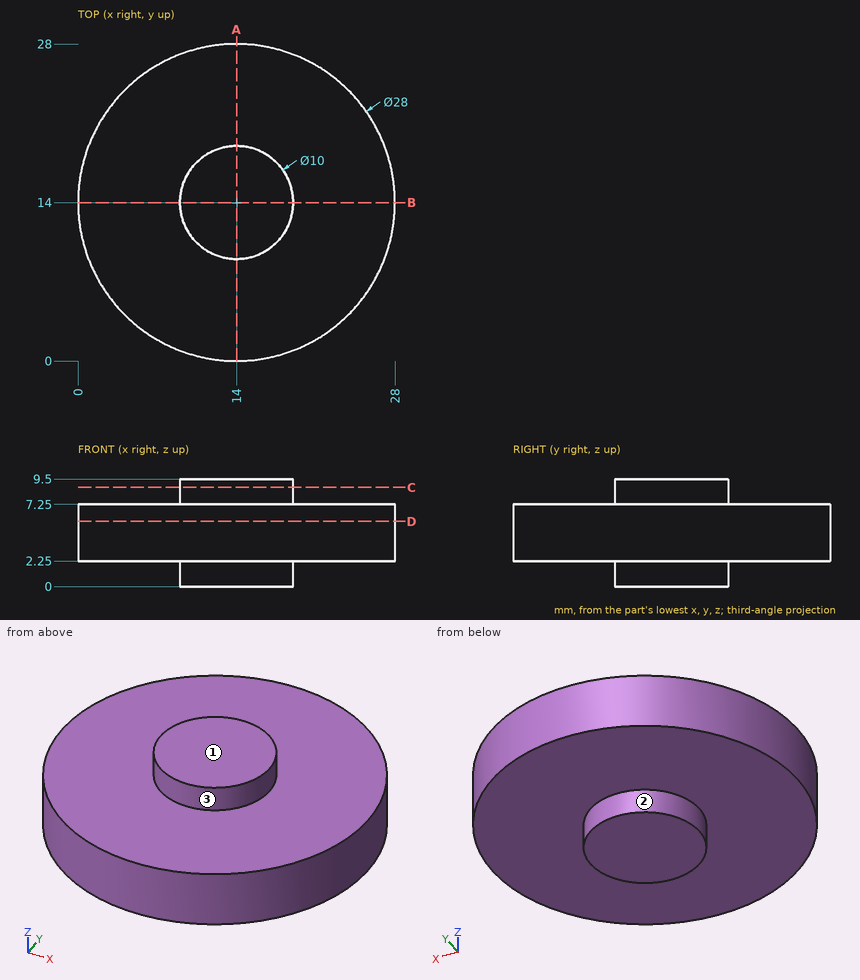
Could you check a few things on this drawing? It's one solid part, dimensions in mm from its lowest x, y, z. A direction names the side the tool comes from. Round coordinates to 2 decimals unless told otherwise and drop trailing zeros. Write each loop counter-clockwise with the first axis right and the second up, starting at its lowest first coordinate (ties: lowest second). Pieces come first, ordered by that corner, then holes.
Q1. Please list where these lines run through material, in increasing order: probe 1 along Z at (x, y) = (9, 11.5); probe 2 along X at (y, z) = (19.5, 6); probe 3 along X at (y, z) = (3, 6).
Q2. If we section it at A-A on x = 14: Write out the boundary of the cut face in (y, z).
Q3. Which directions (+Z, -Z, +X, -X, +Y, -Y) give clear straight access to the entire face, cutting with the end or side of a thin tool? Please do the marked faces 1, 2 and 3.
Q4. Will these pins go through, and if not, where does the flat tip stop? P1, Ø3, axis at y = 5.5, z = 7, coming from the -X side; P2, Ø3, axis at x = 4.5, z = 6.5, coming from the +Y side; P3, Ø4, axis at y = 8.5, z = 7, coming from the +X side.
Q5. If we section it at D-D on z = 5.75: Write out the boundary of the cut face in (x, y), plus the area to 3 significant figures.
Q6. If we section it at C-C on z = 8.75: Write out the boundary of the cut face in (x, y).
Answer below:
1. probe 1: z = 2.25 to 7.25
1. probe 2: x = 1.13 to 26.87
1. probe 3: x = 5.34 to 22.66
2. outline: (0, 2.25) - (9, 2.25) - (9, 0) - (19, 0) - (19, 2.25) - (28, 2.25) - (28, 7.25) - (19, 7.25) - (19, 9.5) - (9, 9.5) - (9, 7.25) - (0, 7.25) - close
3. face 1: +Z, +X, -X, +Y, -Y
3. face 2: -Z
3. face 3: +Z
4. P1: stops at x = 1.88
4. P2: stops at y = 25.49
4. P3: stops at x = 27.56
5. outline: circle Ø28 at (14, 14)
5. area: 616 mm2
6. outline: circle Ø10 at (14, 14)
